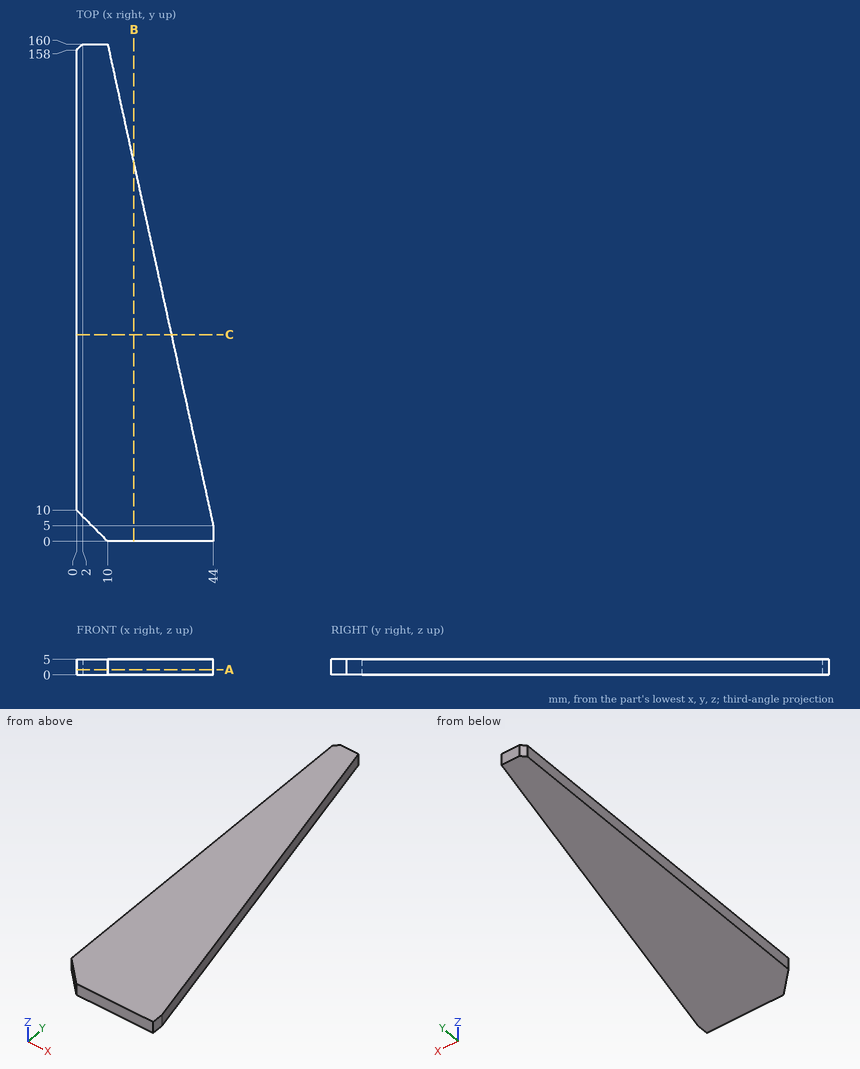
The drawing under review shows one solid part. Ordinate dimensions are in mm from its lowest x, y, z. Round coordinates to 2 decimals unless told otherwise and drop trailing zeros. Loops run counter-clockwise (first coordinate to the right, second up) from the corner with the lowest first, then second, coordinate; pieces in that order, holes last. Notation, with made-up numbers: (3.5, 80) - (33.5, 80) arc R12 ccw to (33.5, 96) - close; hole circle Ø11 at (11.25, 63.5). An arc over 180 degrees is marked (long way). Use a Markdown table: item, result. Add a question column.
Q1. For probe 1 along X at (y, z) = (81, 2.7); probe 2 along X at (y, z) = (76, 2.3); probe 3 along Y at (x, z) = (5.5, 0.95), list the stretches that pass through material, from the lowest coordinate up.
Q2. Add section C-C (y = 66.5). State the section outline as (x, z) points.
Q3. Add section A-A (z = 1.65). State the section outline as (x, y) points, plus the area to 3 significant figures.
Q4. Insertion check: pin 1 Ø6 at (x, y) = (24, 118.5) entering from -Z. The pin has a flat end and moves straight along its axis. Give the tip position at first contact, or say it passes through.
Q5. Add section B-B (x = 18.5). State the section outline as (y, z) points.
Worked answers:
| question | item | result |
|---|---|---|
| 1 | probe 1 | 0 to 27.33 |
| 1 | probe 2 | 0 to 28.43 |
| 1 | probe 3 | 4.5 to 160 |
| 2 | outline | (0, 0) - (30.51, 0) - (30.51, 5) - (0, 5) - close |
| 3 | outline | (0, 10) - (10, 0) - (44, 0) - (44, 5) - (10, 160) - (2, 160) - (0, 158) - close |
| 3 | area | 4,350 mm² |
| 4 | pin 1 | through |
| 5 | outline | (0, 0) - (121.25, 0) - (121.25, 5) - (0, 5) - close |
